Geometry check sheet. Reference: the model listing, model coordinates, mm. A direction names the side the tool comes from. Give positions to 0.01 mm unless a question says otherwise; leave off trailing zeros. Order: outer loops, then holes, each group sorted by start corner. A loop starts at its lowest first (then second) coordinate and runs counter-clockwise, first axis right, second up.
from build123d import *

# Parameters (mm, degrees)
SKETCH1_W                      = 60
SKETCH1_H                      = 299.5
BASE_FLANGE1_DEPTH             = 3
EDGE_FLANGE1_STRIP_W           = 14
EDGE_FLANGE1_STRIP_H           = 3
EDGE_FLANGE1_STRIP_CUT_DEPTH   = 299.5
EDGE_FLANGE1_DEPTH             = 299.5
EDGE_FLANGE2_STRIP_W           = 14
EDGE_FLANGE2_STRIP_H           = 3
EDGE_FLANGE2_STRIP_CUT_DEPTH   = 56
EDGE_FLANGE2_STRIP_2_W         = 14
EDGE_FLANGE2_STRIP_2_H         = 3
EDGE_FLANGE2_STRIP_CUT_2_DEPTH = 56
EDGE_FLANGE2_STRIP_3_W         = 14
EDGE_FLANGE2_STRIP_3_H         = 3
EDGE_FLANGE2_STRIP_CUT_3_DEPTH = 56
EDGE_FLANGE2_STRIP_4_W         = 14
EDGE_FLANGE2_STRIP_4_H         = 3
EDGE_FLANGE2_STRIP_CUT_4_DEPTH = 56
EDGE_FLANGE2_DEPTH             = 56
EDGE_FLANGE2_BEND_DEPTH        = 56
EDGE_FLANGE2_BEND_2_DEPTH      = 56
EDGE_FLANGE2_BEND_3_DEPTH      = 56
SKETCH18_R                     = 4.6
EXTRUDE1_DEPTH                 = 313.712727595
SKETCH19_R                     = 4.6
EXTRUDE2_DEPTH                 = 3
SKETCH20_R                     = 4.6
EXTRUDE3_DEPTH                 = 3


# Sheet-metal steps are written as plain solids
with BuildPart() as part:
    # Sketch1 → Base-Flange1 (new body)
    with BuildSketch(Plane(origin=(0, 0, 0), x_dir=(1, 0, 0), z_dir=(0, 1, 0))):
        Rectangle(SKETCH1_W, SKETCH1_H)
    extrude(amount=BASE_FLANGE1_DEPTH)

    # Edge-Flange1 strip (across the edge) → Edge-Flange1 strip cut (cut)
    with BuildSketch(Plane(origin=(-30, 3, -149.75), x_dir=(1, 0, 0), z_dir=(0, 0, 1))):
        with Locations((-3, -1.5)):
            Rectangle(EDGE_FLANGE1_STRIP_W, EDGE_FLANGE1_STRIP_H)
    extrude(amount=EDGE_FLANGE1_STRIP_CUT_DEPTH, mode=Mode.SUBTRACT)

    # Edge-Flange1 section (across the edge) → Edge-Flange1 (add)
    with BuildSketch(Plane(origin=(-30, 3, -149.75), x_dir=(1, 0, 0), z_dir=(0, 0, 1))):
        with BuildLine():
            Line((0, 1), (0, 57))
            Line((0, 57), (3, 57))
            Line((3, 57), (3, 1))
            ThreePointArc((3, 1), (3.292893219, 0.292893219), (4, 0))
            Line((4, 0), (4, -3))
            ThreePointArc((4, -3), (1.171572875, -1.828427125), (0, 1))
        make_face()
    extrude(amount=EDGE_FLANGE1_DEPTH)

    # Edge-Flange2 strip (across the edge) → Edge-Flange2 strip cut (cut)
    with BuildSketch(Plane(origin=(-30, 4, 149.75), x_dir=(0, 0, -1), z_dir=(0, 1, 0))):
        with Locations((-3, -1.5)):
            Rectangle(EDGE_FLANGE2_STRIP_W, EDGE_FLANGE2_STRIP_H)
    extrude(amount=EDGE_FLANGE2_STRIP_CUT_DEPTH, mode=Mode.SUBTRACT)

    # Edge-Flange2 strip 2 (across the edge) → Edge-Flange2 strip cut 2 (cut)
    with BuildSketch(Plane(origin=(30, 0, 149.75), x_dir=(0, 0, -1), z_dir=(-1, 0, 0))):
        with Locations((-3, -1.5)):
            Rectangle(EDGE_FLANGE2_STRIP_2_W, EDGE_FLANGE2_STRIP_2_H)
    extrude(amount=EDGE_FLANGE2_STRIP_CUT_2_DEPTH, mode=Mode.SUBTRACT)

    # Edge-Flange2 strip 3 (across the edge) → Edge-Flange2 strip cut 3 (cut)
    with BuildSketch(Plane(origin=(-30, 60, -149.75), x_dir=(0, 0, 1), z_dir=(0, -1, 0))):
        with Locations((-3, -1.5)):
            Rectangle(EDGE_FLANGE2_STRIP_3_W, EDGE_FLANGE2_STRIP_3_H)
    extrude(amount=EDGE_FLANGE2_STRIP_CUT_3_DEPTH, mode=Mode.SUBTRACT)

    # Edge-Flange2 strip 4 (across the edge) → Edge-Flange2 strip cut 4 (cut)
    with BuildSketch(Plane(origin=(-26, 0, -149.75), x_dir=(0, 0, 1), z_dir=(1, 0, 0))):
        with Locations((-3, -1.5)):
            Rectangle(EDGE_FLANGE2_STRIP_4_W, EDGE_FLANGE2_STRIP_4_H)
    extrude(amount=EDGE_FLANGE2_STRIP_CUT_4_DEPTH, mode=Mode.SUBTRACT)

    # Edge-Flange2 section (across the edge) → Edge-Flange2 (add)
    with BuildSketch(Plane(origin=(-30, 4, 149.75), x_dir=(0, 0, -1), z_dir=(0, 1, 0))):
        with BuildLine():
            Line((0, 1), (0, 37))
            Line((0, 37), (3, 37))
            Line((3, 37), (3, 1))
            ThreePointArc((3, 1), (3.292893219, 0.292893219), (4, 0))
            Line((4, 0), (4, -3))
            ThreePointArc((4, -3), (1.171572875, -1.828427125), (0, 1))
        make_face()
    extrude(amount=EDGE_FLANGE2_DEPTH)

    # Edge-Flange2 section 2 (across the edge) → Edge-Flange2 bend (add)
    with BuildSketch(Plane(origin=(30, 0, 149.75), x_dir=(0, 0, -1), z_dir=(-1, 0, 0))):
        with BuildLine():
            Line((0, 1), (0, 37))
            Line((0, 37), (3, 37))
            Line((3, 37), (3, 1))
            ThreePointArc((3, 1), (3.292893219, 0.292893219), (4, 0))
            Line((4, 0), (4, -3))
            ThreePointArc((4, -3), (1.171572875, -1.828427125), (0, 1))
        make_face()
    extrude(amount=EDGE_FLANGE2_BEND_DEPTH)

    # Edge-Flange2 section 3 (across the edge) → Edge-Flange2 bend 2 (add)
    with BuildSketch(Plane(origin=(-30, 60, -149.75), x_dir=(0, 0, 1), z_dir=(0, -1, 0))):
        with BuildLine():
            Line((0, 1), (0, 37))
            Line((0, 37), (3, 37))
            Line((3, 37), (3, 1))
            ThreePointArc((3, 1), (3.292893219, 0.292893219), (4, 0))
            Line((4, 0), (4, -3))
            ThreePointArc((4, -3), (1.171572875, -1.828427125), (0, 1))
        make_face()
    extrude(amount=EDGE_FLANGE2_BEND_2_DEPTH)

    # Edge-Flange2 section 4 (across the edge) → Edge-Flange2 bend 3 (add)
    with BuildSketch(Plane(origin=(-26, 0, -149.75), x_dir=(0, 0, 1), z_dir=(1, 0, 0))):
        with BuildLine():
            Line((0, 1), (0, 37))
            Line((0, 37), (3, 37))
            Line((3, 37), (3, 1))
            ThreePointArc((3, 1), (3.292893219, 0.292893219), (4, 0))
            Line((4, 0), (4, -3))
            ThreePointArc((4, -3), (1.171572875, -1.828427125), (0, 1))
        make_face()
    extrude(amount=EDGE_FLANGE2_BEND_3_DEPTH)

    # Sketch18 → Extrude1 (cut, through all)
    with BuildSketch(Plane.XY.offset(149.75)):
        with Locations((-47, 47.5)):
            Circle(SKETCH18_R)
        with Locations((-47, 17.5)):
            Circle(SKETCH18_R)
        with Locations((-12.5, -17)):
            Circle(SKETCH18_R)
        with Locations((17.5, -17)):
            Circle(SKETCH18_R)
    extrude(amount=-EXTRUDE1_DEPTH, mode=Mode.SUBTRACT)

    # Sketch19 → Extrude2 (cut)
    with BuildSketch(Plane(origin=(-27, 0, 0), x_dir=(0, 0, -1), z_dir=(1, 0, 0))):
        with Locations(Location((-99.75, 35, 0), (0, 0, 90))):
            Circle(SKETCH19_R)
        with Locations(Location((69.75, 35, 0), (0, 0, 90))):
            Circle(SKETCH19_R)
    extrude(amount=-EXTRUDE2_DEPTH, mode=Mode.SUBTRACT)

    # Sketch20 → Extrude3 (cut)
    with BuildSketch(Plane(origin=(0, 3, 0), x_dir=(1, 0, 0), z_dir=(0, 1, 0))):
        with Locations(Location((5, 69.75, 0), (0, 0, 270))):
            Circle(SKETCH20_R)
        with Locations(Location((5, -99.75, 0), (0, 0, 270))):
            Circle(SKETCH20_R)
    extrude(amount=-EXTRUDE3_DEPTH, mode=Mode.SUBTRACT)


solid = part.part
Item 1: Sectioned sample at C-C (z = 99.75). Enter the section's corners in (x, y).
Reported:
outline: (-30, 4) arc R4 ccw to (-26, 0) - (0.4, 0) - (0.4, 3) - (-26, 3) arc R1 cw to (-27, 4) - (-27, 30.4) - (-30, 30.4) - close; (-30, 39.6) - (-27, 39.6) - (-27, 60) - (-30, 60) - close; (9.6, 0) - (30, 0) - (30, 3) - (9.6, 3) - close
Item 2: Sectioned sample at B-B (x = 17.5). Enter the section's corners in (y, z).
Reported:
outline: (-37, -149.75) - (-21.6, -149.75) - (-21.6, -146.75) - (-37, -146.75) - close; (-37, 146.75) - (-21.6, 146.75) - (-21.6, 149.75) - (-37, 149.75) - close; (-12.4, -149.75) - (-1, -149.75) arc R4 ccw to (3, -145.75) - (3, 145.75) arc R4 ccw to (-1, 149.75) - (-12.4, 149.75) - (-12.4, 146.75) - (-1, 146.75) arc R1 cw to (0, 145.75) - (0, -145.75) arc R1 cw to (-1, -146.75) - (-12.4, -146.75) - close
Item 3: Sectioned sample at D-D (y = -17). Enter the section's corners in (x, z).
Reported:
outline: (-26, -149.75) - (-17.1, -149.75) - (-17.1, -146.75) - (-26, -146.75) - close; (-26, 146.75) - (-17.1, 146.75) - (-17.1, 149.75) - (-26, 149.75) - close; (-7.9, -149.75) - (12.9, -149.75) - (12.9, -146.75) - (-7.9, -146.75) - close; (-7.9, 146.75) - (12.9, 146.75) - (12.9, 149.75) - (-7.9, 149.75) - close; (22.1, -149.75) - (30, -149.75) - (30, -146.75) - (22.1, -146.75) - close; (22.1, 146.75) - (30, 146.75) - (30, 149.75) - (22.1, 149.75) - close
Item 4: Set-up check for faces 4 (the flat face through (-27, 32, -2)), 5 (the cylindrical face through (-13.1, -12.44, -148.23)), 6 (the flat face through (2, -19, 146.75)), 7 (the flat face through (-30, 32, -2)): record each of +Z, -Z, +X, -X, +Y, -Y from which the full face is reachable in a straight line by a thin tool's end or side.
Reported:
face 4: +Z, -Z, +X, +Y
face 5: +Z, -Z
face 6: +X, -X, -Y
face 7: -X, +Y, -Y
Item 5: Scan lines: L1, parallel to Z at x = 11, y = -12; L2, parallel to Y at x = -16, z = 15; L3, parallel to X at y = 30, z = -45.5. Record each from-to range of solid material in increasing order.
Reported:
L1: z = -149.75 to -146.75, 146.75 to 149.75
L2: y = 0 to 3
L3: x = -30 to -27
Item 6: Gauge pin test, flat ends, axial feed: pin 1 (1.2 mm diameter, centred on x = -48, z = -147, fed in from -Y); pin 2 (8 mm diameter, centred on x = 11.5, z = 26, fed in from -Y); pin 3 (17 mm diameter, centred on x = -3.5, z = 10.5, fed in from +Y). Record the tip position at first contact, or that the pin passes through.
Reported:
pin 1: stops at y = 4
pin 2: stops at y = 0
pin 3: stops at y = 3
Item 7: Draft check along X on faces 1 (the cylindrical face through (-28.479, 37.123, -73.831)), 2 (the cylindrical face through (-44.53, 21.38, -148.23)), 3 (the flat face through (30, 1, 1)). Enter one of: released by +X, released by -X, zero draft, split by the parting line, or undercut.
Reported:
face 1: zero draft
face 2: undercut
face 3: released by +X
Item 8: Sectioned sample at A-A (y = -31). Enter the section's corners in (x, z).
Reported:
outline: (-26, -149.75) - (30, -149.75) - (30, -146.75) - (-26, -146.75) - close; (-26, 146.75) - (30, 146.75) - (30, 149.75) - (-26, 149.75) - close
